Autodesk Inventor part; units mm, degrees
ref_plane "a_XY" through (-12.7, 0, 0) normal (1, 0, 0) x (0, 0, -1)
ref_plane "a_YZ" through (-12.7, 0, 0) normal (0, 0, -1) x (0, 1, 0)
ref_plane "a_ZX" through (-12.7, 0, 0) normal (0, 1, 0) x (1, 0, 0)
sketch "Sketch_1" plane through (0, 0, 0) normal (0, 0, 1) x (1, 0, 0)
  line L0 (164.2872, 0) -> (0, 0)
  line L1 (0, 0) -> (0, 3.175)
  line L2 (0, 3.175) -> (164.2872, 3.175)
  line L3 (164.2872, 3.175) -> (164.2872, 0)
  line L4 (164.2872, 0) -> (0, 0)
revolve "Revolution1" add sketch "Sketch_1" angle 360 about axis through (164.2872, 0, 0) along (1, 0, 0)
sketch "Sketch_3" plane through (0, 0, 0) normal (0, 0, 1) x (1, 0, 0)
  line L0 (164.2872, 0) -> (142.113, 0)
  line L1 (142.113, 0) -> (142.113, 9.525)
  line L2 (142.113, 9.525) -> (164.2872, 9.525)
  line L3 (164.2872, 9.525) -> (164.2872, 0)
  line L4 (164.2872, 0) -> (142.113, 0)
revolve "Revolution2" add sketch "Sketch_3" angle 360 about axis through (164.2872, 0, 0) along (1, 0, 0)
sketch "Sketch_4" plane through (0, 0, 0) normal (0, 0, 1) x (1, 0, 0)
  line L0 (0, 0) -> (-12.7, 0)
  line L1 (-12.7, 0) -> (-12.7, 2.634)
  line L2 (-12.7, 2.634) -> (-12.159, 3.175)
  line L3 (-12.159, 3.175) -> (0, 3.175)
  line L4 (0, 3.175) -> (0, 0)
  line L5 (0, 0) -> (-12.7, 0)
revolve "Revolution3" add sketch "Sketch_4" angle 360 about axis through (0, 0, 0) along (1, 0, 0)
ref_plane "a_XY" through (-12.7, 0, 0) normal (1, 0, 0) x (0, 0, -1)
ref_plane "a_YZ" through (-12.7, 0, 0) normal (0, 0, -1) x (0, 1, 0)
ref_plane "a_ZX" through (-12.7, 0, 0) normal (0, 1, 0) x (1, 0, 0)
ref_plane "c1_XY" through (0, 0, 0) normal (1, 0, 0) x (0, 0, -1)
ref_plane "c1_YZ" through (0, 0, 0) normal (0, 0, -1) x (0, 1, 0)
ref_plane "c1_ZX" through (0, 0, 0) normal (0, 1, 0) x (1, 0, 0)
ref_plane "cc1_XY" through (0, 0, -3.175) normal (1, 0, 0) x (0, 0, -1)
ref_plane "cc1_YZ" through (0, 0, -3.175) normal (0, 0, -1) x (0, 1, 0)
ref_plane "cc1_ZX" through (0, 0, -3.175) normal (0, 1, 0) x (1, 0, 0)
ref_plane "cc2_XY" through (0, 0, 3.175) normal (1, 0, 0) x (0, 0, -1)
ref_plane "cc2_YZ" through (0, 0, 3.175) normal (0, 0, -1) x (0, 1, 0)
ref_plane "cc2_ZX" through (0, 0, 3.175) normal (0, 1, 0) x (1, 0, 0)
ref_plane "kk_XY" through (-6.35, 0, 3.175) normal (1, 0, 0) x (0, 0, -1)
ref_plane "kk_YZ" through (-6.35, 0, 3.175) normal (0, 0, -1) x (0, 1, 0)
ref_plane "kk_ZX" through (-6.35, 0, 3.175) normal (0, 1, 0) x (1, 0, 0)
ref_plane "rod_XY" through (164.2872, 0, 0) normal (1, 0, 0) x (0, 0, -1)
ref_plane "rod_YZ" through (164.2872, 0, 0) normal (0, 0, -1) x (0, 1, 0)
ref_plane "rod_ZX" through (164.2872, 0, 0) normal (0, 1, 0) x (1, 0, 0)
properties part number "6.4680.8730.50.500Double acting_00_006.4680.500.75N"
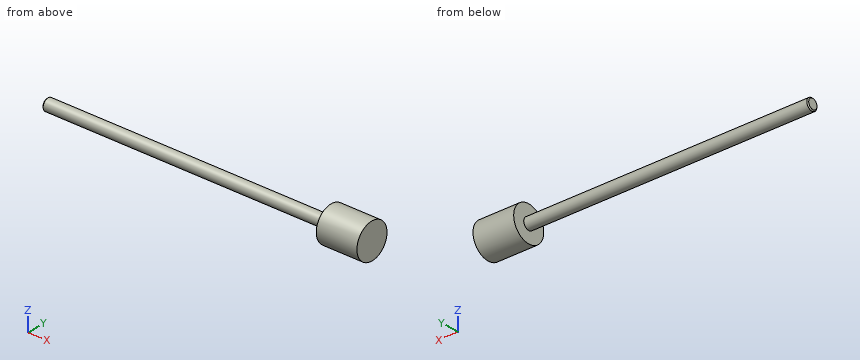
Could you check a few things on this model? Use its own coordinates, in mm. Give positions to 0.01 mm unless a question says otherwise; leave off trailing zeros. Loops run counter-clockwise (first coordinate to the right, second up) from the corner with the lowest first, then second, coordinate; pieces in that order, holes last. Notation, with made-up numbers: (56, 17.5) -> (96, 17.5) arc R14 cw to (96, 40.5) -> close; hole circle Ø8 at (-24.75, 28). An arc over 180 degrees is marked (long way). Answer as CSV lines item,"result". Start each with the question number.
(1) If we section it at C-C on x = 75: Write out the boundary of the cut face in (y, z) (3 decimals), then the cut area to 3 significant figures.
(2) If we section it at D-D on y = 7.5: Write out the boundary of the cut face in (x, z).
(3) If we section it at A-A on y = 0: Write out the boundary of the cut face in (x, z) (3 decimals), then the cut area to 3 significant figures.
(4) I'm going to push flat-ended pins straight in: pin 1 Ø4 at (x, z) = (107.5, 7) entering from +Y; pin 2 Ø9.5 at (y, z) = (-1, 4.5) entering from -X; pin 3 Ø2 at (x, z) = (113, -3) entering from +Y. Where does each tip first touch, or does it pass through?
(5) I need wall thicknesses on probe 1 along X at (y, z) = (-1.25, 6.25); probe 2 along Z at (x, y) = (127, 0) (3 decimals); probe 3 along Y at (x, z) = (21, 0.25). Which ranges of each line are inside material? Lowest first, please.
Computed:
1,outline,"circle Ø6.35 at (0, 0)"
1,area,"31.7 mm2"
2,outline,"(142.11, -5.87) -> (164.29, -5.87) -> (164.29, 5.87) -> (142.11, 5.87) -> close"
3,outline,"(-12.7, -2.634) -> (-12.159, -3.175) -> (142.113, -3.175) -> (142.113, -9.525) -> (164.287, -9.525) -> (164.287, 9.525) -> (142.113, 9.525) -> (142.113, 3.175) -> (-12.159, 3.175) -> (-12.7, 2.634) -> close"
3,area,"1,410 mm2"
4,pin 1,"passes through"
4,pin 2,"stops at x = -12.7"
4,pin 3,"stops at y = 2.47"
5,probe 1,"x = 142.11 to 164.29"
5,probe 2,"z = -3.175 to 3.175"
5,probe 3,"y = -3.17 to 3.17"
